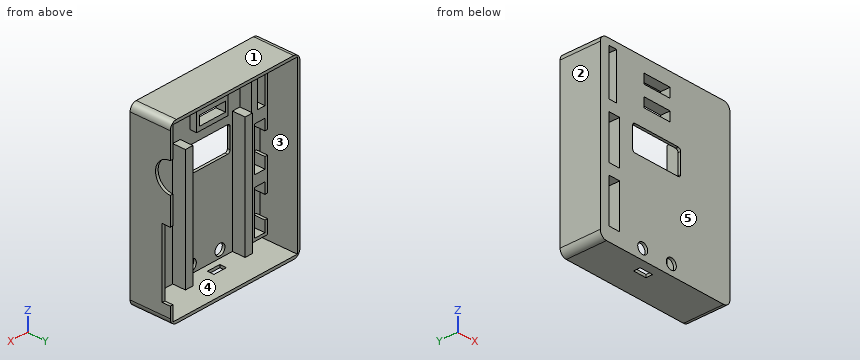
from build123d import *

# Parameters (mm, degrees)
F0_W      = 100
F0_H      = 125
F0_W_2    = 8.5
F0_H_2    = 32.25
F0_R      = 4
F0_R_2    = 2.75
F0_R_3    = 2
F0_W_3    = 6
F0_H_3    = 34
F0_W_4    = 21
F0_H_4    = 7
F1_DEPTH  = 2
F2_W      = 6
F2_H      = 89
F3_DEPTH  = 8.5
F5_DEPTH  = 8.5
F6_W      = 6
F6_H      = 34
F7_DEPTH  = 8.5
F8_W      = 21
F8_H      = 7
F9_DEPTH  = 5
F10_W     = 104.2
F10_H     = 129.2
F10_W_2   = 100
F10_H_2   = 125
F11_DEPTH = 30
F12_R     = 11
F12_W     = 12
F12_H     = 50
F13_DEPTH = 5
F14_R     = 3.75
F15_DEPTH = 1
F16_W     = 6
F16_H     = 89
F17_DEPTH = 1
F18_W     = 6
F18_H     = 89
F19_DEPTH = 1
F20_W     = 10
F20_H     = 5
F21_DEPTH = 5
F22_R     = 5
F23_W     = 38.6
F23_H     = 18.75
F23_R     = 2.75
F23_R_2   = 2
F24_DEPTH = 25
F25_R     = 2


with BuildPart() as f1:
    # F0 (on Front) → F1 (new body)
    with BuildSketch(Plane.XZ):
        with Locations((50, -62.5)):
            Rectangle(F0_W, F0_H)
        with Locations((9.25, -100.875)):
            Rectangle(F0_W_2, F0_H_2, mode=Mode.SUBTRACT)
        with Locations((32, -119.5)):
            Circle(F0_R, mode=Mode.SUBTRACT)
        with Locations((55, -119.5)):
            Circle(F0_R, mode=Mode.SUBTRACT)
        with Locations((9.25, -60.625)):
            Rectangle(F0_W_2, F0_H_2, mode=Mode.SUBTRACT)
        with Locations((34, -56)):
            Circle(F0_R_2, mode=Mode.SUBTRACT)
        with Locations((27.5, -47)):
            Circle(F0_R_3, mode=Mode.SUBTRACT)
        with Locations((8, -19.5)):
            Rectangle(F0_W_3, F0_H_3, mode=Mode.SUBTRACT)
        with Locations((43.5, -26.5)):
            Rectangle(F0_W_4, F0_H_4, mode=Mode.SUBTRACT)
        with Locations((43.5, -11.5)):
            Rectangle(F0_W_4, F0_H_4, mode=Mode.SUBTRACT)
        with Locations((52, -56)):
            Circle(F0_R_2, mode=Mode.SUBTRACT)
        with Locations((58.5, -47)):
            Circle(F0_R_3, mode=Mode.SUBTRACT)
    extrude(amount=F1_DEPTH)

    # F2 (on face) → F3 (join)
    with BuildSketch(Plane(origin=(0, 0, 0), x_dir=(-1, 0, 0), z_dir=(0, 1, 0))):
        Polygon((-22, -125), (-16, -125), (-16, -117), (-16, -36), (-22, -36), align=None)
        with Locations((-67, -80.5)):
            Rectangle(F2_W, F2_H)
    extrude(amount=F3_DEPTH)

    # F4 (on face) → F5 (join)
    with BuildSketch(Plane(origin=(0, 0, 0), x_dir=(-1, 0, 0), z_dir=(0, 1, 0))):
        Polygon((-16, -119.1), (-5, -119.1), (-2.9, -119.1), (-2.9, -109), (-5, -109), (-5, -117), (-13.5, -117), (-13.5, -84.75), (-5, -84.75), (-5, -92.75), (-2.9, -92.75), (-2.9, -82.65), (-5, -82.65), (-16, -82.65), align=None)
        Polygon((-16, -78.85), (-16, -82.65), (-5, -82.65), (-2.9, -82.65), (-2.9, -78.85), (-5, -78.85), align=None)
        Polygon((-16, -42.4), (-16, -78.85), (-5, -78.85), (-2.9, -78.85), (-2.9, -68.75), (-5, -68.75), (-5, -76.75), (-13.5, -76.75), (-13.5, -44.5), (-5, -44.5), (-5, -52.5), (-2.9, -52.5), (-2.9, -42.4), align=None)
    extrude(amount=F5_DEPTH)

    # F6 (on face) → F7 (join)
    with BuildSketch(Plane(origin=(0, 0, 0), x_dir=(-1, 0, 0), z_dir=(0, 1, 0))):
        Polygon((-2.9, -38.6), (-5, -38.6), (-16, -38.6), (-16, -42.4), (-2.9, -42.4), align=None)
        Polygon((-16, -38.6), (-5, -38.6), (-2.9, -38.6), (-2.9, -0.4), (-16, -0.4), align=None)
        with Locations((-8, -19.5)):
            Rectangle(F6_W, F6_H, mode=Mode.SUBTRACT)
    extrude(amount=F7_DEPTH)

    # F8 (on face) → F9 (join)
    with BuildSketch(Plane(origin=(0, 0, 0), x_dir=(-1, 0, 0), z_dir=(0, 1, 0))):
        Polygon((-56.1, -33.1), (-54, -33.1), (-30.9, -33.1), (-30.9, -19.9), (-56.1, -19.9), align=None)
        with Locations((-43.5, -26.5)):
            Rectangle(F8_W, F8_H, mode=Mode.SUBTRACT)
        Polygon((-56.1, -18.1), (-56.1, -19.9), (-30.9, -19.9), (-30.9, -18.1), (-54, -18.1), align=None)
        Polygon((-56.1, -4.9), (-56.1, -18.1), (-54, -18.1), (-30.9, -18.1), (-30.9, -4.9), align=None)
        with Locations((-43.5, -11.5)):
            Rectangle(F8_W, F8_H, mode=Mode.SUBTRACT)
    extrude(amount=F9_DEPTH)

    # F10 (on face) → F11 (join)
    with BuildSketch(Plane.XZ.offset(2)):
        with Locations((50, -62.5)):
            Rectangle(F10_W, F10_H)
        with Locations((50, -62.5)):
            Rectangle(F10_W_2, F10_H_2, mode=Mode.SUBTRACT)
    extrude(amount=-F11_DEPTH)

    # F12 (on face) → F13 (cut)
    with BuildSketch(Plane.YZ.offset(102.1)):
        with Locations((28, -32.9)):
            Circle(F12_R)
        with Locations((28, -89.1)):
            Rectangle(F12_W, F12_H)
    extrude(amount=-F13_DEPTH, mode=Mode.SUBTRACT)

    # F14 (on face) → F15 (cut)
    with BuildSketch(Plane(origin=(0, 0, 0), x_dir=(-1, 0, 0), z_dir=(0, 1, 0))):
        with Locations((-34, -56)):
            Circle(F14_R)
        with Locations((-52, -56)):
            Circle(F14_R)
    extrude(amount=-F15_DEPTH, mode=Mode.SUBTRACT)

    # F16 (on face) → F17 (join)
    with BuildSketch(Plane(origin=(0, 8.5, 0), x_dir=(-1, 0, 0), z_dir=(0, 1, 0))):
        with Locations((-19, -80.5)):
            Rectangle(F16_W, F16_H)
    extrude(amount=F17_DEPTH)

    # F18 (on face) → F19 (join)
    with BuildSketch(Plane(origin=(0, 8.5, 0), x_dir=(-1, 0, 0), z_dir=(0, 1, 0))):
        with Locations((-67, -80.5)):
            Rectangle(F18_W, F18_H)
    extrude(amount=F19_DEPTH)

    # F20 (on face) → F21 (cut)
    with BuildSketch(Plane.XY.offset(-125)):
        with Locations((42, 7)):
            Rectangle(F20_W, F20_H)
    extrude(amount=-F21_DEPTH, mode=Mode.SUBTRACT)

    # F22
    f22_edges = [f1.edges().sort_by_distance(p)[0] for p in [
        (102.1, 13, 2.1),
        (-2.1, 13, 2.1),
        (-2.1, 13, -127.1),
        (102.1, 13, -127.1),
    ]]
    fillet(f22_edges, radius=F22_R)

    # F23 (on face) → F24 (cut)
    with BuildSketch(Plane.XZ.offset(2)):
        with Locations((43.2, -52.375)):
            Rectangle(F23_W, F23_H)
        with Locations((34, -56)):
            Circle(F23_R, mode=Mode.SUBTRACT)
        with Locations((27.5, -47)):
            Circle(F23_R_2, mode=Mode.SUBTRACT)
        with Locations((52, -56)):
            Circle(F23_R, mode=Mode.SUBTRACT)
        with Locations((58.5, -47)):
            Circle(F23_R_2, mode=Mode.SUBTRACT)
    extrude(amount=-F24_DEPTH, mode=Mode.SUBTRACT)

    # F25
    f25_edges = [f1.edges().sort_by_distance(p)[0] for p in [
        (23.9, -1, -43),
        (62.5, -1, -43),
        (23.9, -1, -61.75),
        (62.5, -1, -61.75),
    ]]
    fillet(f25_edges, radius=F25_R)


solid = f1.part
Check sheet for the modelled part. Datum: model origin and axes. Units: mm. Face numbers are marked on the shaded views. A direction names the side the tool comes from. Round coordinates to 2 decimals unless told otherwise and drop trailing zeros. Write each loop counter-clockwise with the first axis right and the second up, starting at its lowest first coordinate (ties: lowest second). Pieces come first, ordered by that corner, then holes. Notation, with made-up numbers: (87, 43) -> (101, 43) arc R20 cw to (101, 80) -> close; hole circle Ø4 at (-19.5, 15.5). An arc over 180 degrees is marked (long way). Answer as CSV lines item,"result". Start each with the question number.
1) Release check for a two-part mould opening along X. For the marked faces 1, 2 and 3 record: pulls with the +X half, pulls with the -X half, needs draft (parallel to the pull), parting line crosses it, or undercut.
2) Section check A-A on z = -13.5. Enter the section's corners in (x, y).
3) Go/stop test with flat-tipped pins: P1, Ø6.5, axis at x = 66.5, z = -71, coming from the +Y side; P2, Ø1.5, axis at x = 44, z = -12.5, coming from the -Y side. Record where each tip stops, or that it passes through.
4) Section check B-B on y = 14. Enter the section's corners in (x, z), and give its area (3 significant figures).
5) Section check C-C on z = -48. Enter the section's corners in (x, y), and give its area (3 significant figures).
6) Section check D-D on y = 25.5. Enter the section's corners in (x, z), and give its area (3 significant figures).
7) Material ranges on line 1 (Z direction, x = 55, y = -1.3); line 2 (Z direction, x = 55.5, y = 2.5); line 3 (X direction, y = 5.75, z = -42.5), recorded low to high. Write a range as from..to.
8) Tool access check on the marked faces 4 and 5. Record the directions out of +Z, -Z, +X, -X, +Y, -Y that give a thin tool (end or side, any length) a straight path to the whole face; none if there is none.
Found:
1,face 1,"needs draft"
1,face 2,"pulls with the -X half"
1,face 3,"undercut"
2,outline,"(-2.1, -2) -> (5, -2) -> (5, 8.5) -> (2.9, 8.5) -> (2.9, 0) -> (0, 0) -> (0, 28) -> (-2.1, 28) -> close; (11, -2) -> (33, -2) -> (33, 5) -> (30.9, 5) -> (30.9, 0) -> (16, 0) -> (16, 8.5) -> (11, 8.5) -> close; (54, -2) -> (102.1, -2) -> (102.1, 28) -> (100, 28) -> (100, 0) -> (56.1, 0) -> (56.1, 5) -> (54, 5) -> close"
3,P1,"stops at y = 9.5"
3,P2,"passes through"
4,outline,"(-2.1, -122.1) arc R5 ccw to (2.9, -127.1) -> (97.1, -127.1) arc R5 ccw to (102.1, -122.1) -> (102.1, -2.9) arc R5 ccw to (97.1, 2.1) -> (2.9, 2.1) arc R5 ccw to (-2.1, -2.9) -> close; hole (0, -125) -> (100, -125) -> (100, 0) -> (0, 0) -> close"
4,area,"941 mm^2"
5,outline,"(-2.1, -2) -> (5, -2) -> (5, 8.5) -> (2.9, 8.5) -> (2.9, 0) -> (0, 0) -> (0, 28) -> (-2.1, 28) -> close; (13.5, -2) -> (23.9, -2) -> (23.9, 0) -> (22, 0) -> (22, 9.5) -> (16, 9.5) -> (16, 8.5) -> (13.5, 8.5) -> close; (62.5, -2) -> (102.1, -2) -> (102.1, 28) -> (100, 28) -> (100, 0) -> (70, 0) -> (70, 9.5) -> (64, 9.5) -> (64, 0) -> (62.5, 0) -> close"
5,area,"385 mm^2"
6,outline,"(-2.1, -122.1) arc R5 ccw to (2.9, -127.1) -> (97.1, -127.1) arc R5 ccw to (102.1, -122.1) -> (102.1, -114.1) -> (100, -114.1) -> (100, -125) -> (0, -125) -> (0, 0) -> (100, 0) -> (100, -22.19) -> (102.1, -22.19) -> (102.1, -2.9) arc R5 ccw to (97.1, 2.1) -> (2.9, 2.1) arc R5 ccw to (-2.1, -2.9) -> close; (100, -64.1) -> (102.1, -64.1) -> (102.1, -43.61) -> (100, -43.61) -> close"
6,area,"791 mm^2"
7,line 1,"z = -127.1..-123.5, -115.5..-61.75, -43..2.1"
7,line 2,"z = -127.1..-125, -33.1..-4.9, 0..2.1"
7,line 3,"x = -2.1..0, 2.9..22, 64..70, 100..102.1"
8,face 4,"+Y"
8,face 5,"+Z, -Z, +X, -X, -Y"
